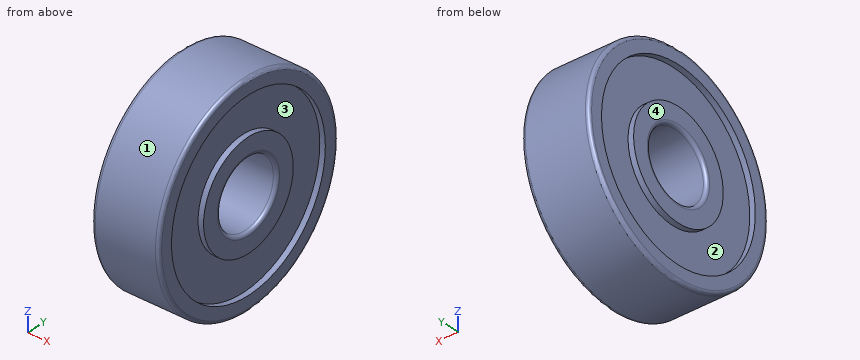
```python
from build123d import *

# Parameters (mm, degrees)
FILLET1_R = 0.3
FILLET2_R = 0.3


with BuildPart() as part:
    # Sketch1 → Revolve1 (revolve)
    with BuildSketch(Plane.XY):
        Polygon((0, 3), (6, 3), (6, 4.75), (5.5, 4.75), (5.5, 8.15), (6, 8.15), (6, 9.5), (0, 9.5), (0, 8.15), (0.5, 8.15), (0.5, 4.75), (0, 4.75), align=None)
    revolve(axis=Axis((0, 0, 0), (1, 0, 0)))

    # Fillet1
    fillet1_edges = [part.edges().sort_by_distance(p)[0] for p in [
        (0, -9.5, 0),
        (6, -9.5, 0),
    ]]
    fillet(fillet1_edges, radius=FILLET1_R)

    # Fillet2
    fillet2_edges = [part.edges().sort_by_distance(p)[0] for p in [
        (6, -3, 0),
        (0, -3, 0),
    ]]
    fillet(fillet2_edges, radius=FILLET2_R)


solid = part.part
```
Read the model definition and answer for the solid it produces. Units are mm, in the model's axes. Face numbers are marked on the shaded views. Round coordinates to 2 decimals unless told otherwise and drop trailing zeros. Loops run counter-clockwise (first coordinate to the right, second up) from the corner with the lowest first, then second, coordinate; pieces in that order, holes last. Notation, with made-up numbers: (84, -2) -> (91, -2) arc R21 cw to (91, 25) -> close; hole circle Ø9 at (-6.5, 39.25). An arc over 180 degrees is marked (long way). One line per item, written item: value.
1) A cutting plane is placed at C-C (x = 2.9). Determine the outline of the cut face in (y, z), and give its area (3 significant figures).
Answer list:
outline: circle Ø19 at (0, 0); hole circle Ø6 at (0, 0)
area: 255 mm²
2) The mould has two halves that part along Y. Classify the marked faces 1, 2, 3 and 4: pulls with the +Y half, pulls with the -Y half, needs draft (parallel to the pull), parting line crosses it, or undercut.
Answer list:
face 1: parting line crosses it
face 2: undercut
face 3: undercut
face 4: needs draft
3) Consider L1, parallel to Z at x = 0.25, y = 0; L2, parallel to Z at x = 2.2, y = 0; L3, parallel to X at y = 0.5, z = -5.25. Determine where each line is inside the solid, lowest interval first. Write a range as [from, to].
Answer list:
L1: z = [-9.5, -8.15], [-4.75, -3], [3, 4.75], [8.15, 9.5]
L2: z = [-9.5, -3], [3, 9.5]
L3: x = [0.5, 5.5]
4) A flat-ended cylindrical pin translates along its axis: P1, Ø5.5, axis at y = 0, z = 0, coming from the -X side. Find the tip coordinate at first contact, or state that the pin passes through.
Answer list:
P1: passes through
